Geometry: final body of the model. Coordinates: model frame, mm. A direction names the side the tool comes from. Give positions to 0.01 mm unless a question says otherwise; leave off trailing zeros. Loops run counter-clockwise (first coordinate to the right, second up) from the corner with the lowest first, then second, coordinate; pieces in that order, holes last. Notation, with made-up numbers: (-9, -27.75) - (23, -27.75) arc R16 ccw to (23, -15.75) - close; hole circle Ø3 at (77, 53.5). An arc over 180 degrees is marked (long way). Answer in a Markdown table with one row per item.
from build123d import *

# Parameters (mm, degrees)
EXTRUDE_1_DEPTH     = 2.5
SKETCH_2_R          = 1.6
CUT_EXTRUDE_1_DEPTH = 139.744369255
SKETCH_3_R          = 1.05
CUT_EXTRUDE_2_DEPTH = 139.744369255
SKETCH_4_R          = 1.1
SKETCH_4_R_2        = 15
SKETCH_4_R_3        = 6
CUT_EXTRUDE_3_DEPTH = 139.744369255
CHAMFER_1_SIZE      = 1
CHAMFER_2_SIZE      = 1


with BuildPart() as part:
    # 草图1 → 凸台-拉伸1 (new, symmetric)
    with BuildSketch(Plane.XY):
        with BuildLine():
            Line((-125, 29), (-125, 20))
            ThreePointArc((-125, 20), (-123.535533906, 16.464466094), (-120, 15))
            Line((-120, 15), (-98, 15))
            ThreePointArc((-98, 15), (-94.464466094, 13.535533906), (-93, 10))
            Line((-93, 10), (-93, -10))
            ThreePointArc((-93, -10), (-94.464466094, -13.535533906), (-98, -15))
            Line((-98, -15), (-120, -15))
            ThreePointArc((-120, -15), (-123.535533906, -16.464466094), (-125, -20))
            Line((-125, -20), (-125, -29))
            ThreePointArc((-125, -29), (-124.906679931, -29.9615051), (-124.630203177, -30.88711911))
            Line((-124.630203177, -30.88711911), (-118.51669464, -45.88711911))
            ThreePointArc((-118.51669464, -45.88711911), (-99.99588193, -58.338642669), (-81.475069221, -45.88711911))
            Line((-81.475069221, -45.88711911), (-75.361560684, -30.88711911))
            ThreePointArc((-75.361560684, -30.88711911), (-74.837036555, -30.24239728), (-74.04203004, -30))
            Line((-74.04203004, -30), (-1.339745962, -30))
            ThreePointArc((-1.339745962, -30), (-0.045650737, -30.170370869), (1.160254038, -30.669872981))
            Line((1.160254038, -30.669872981), (50.801270189, -59.330127019))
            ThreePointArc((50.801270189, -59.330127019), (52.007174964, -59.829629131), (53.301270189, -60))
            Line((53.301270189, -60), (95, -60))
            ThreePointArc((95, -60), (98.535533906, -58.535533906), (100, -55))
            Line((100, -55), (100, -32.886751346))
            ThreePointArc((100, -32.886751346), (99.330127019, -30.386751346), (97.5, -28.556624327))
            Line((97.5, -28.556624327), (55.538475773, -4.330127019))
            ThreePointArc((55.538475773, -4.330127019), (53.038475773, 0), (55.538475773, 4.330127019))
            Line((55.538475773, 4.330127019), (97.5, 28.556624327))
            ThreePointArc((97.5, 28.556624327), (99.330127019, 30.386751346), (100, 32.886751346))
            Line((100, 32.886751346), (100, 55))
            ThreePointArc((100, 55), (98.535533906, 58.535533906), (95, 60))
            Line((95, 60), (53.301270189, 60))
            ThreePointArc((53.301270189, 60), (52.007174964, 59.829629131), (50.801270189, 59.330127019))
            Line((50.801270189, 59.330127019), (0, 30))
            Line((0, 30), (-74.04203004, 30))
            ThreePointArc((-74.04203004, 30), (-74.837036555, 30.24239728), (-75.361560684, 30.88711911))
            Line((-75.361560684, 30.88711911), (-81.475069221, 45.88711911))
            ThreePointArc((-81.475069221, 45.88711911), (-99.99588193, 58.338642669), (-118.51669464, 45.88711911))
            Line((-118.51669464, 45.88711911), (-124.630203177, 30.88711911))
            ThreePointArc((-124.630203177, 30.88711911), (-124.906679931, 29.9615051), (-125, 29))
        make_face()
    extrude(amount=EXTRUDE_1_DEPTH, both=True)

    # 草图2 → 切除-拉伸1 (cut, through all)
    with BuildSketch(Plane.XY.offset(2.5)):
        with Locations((-104.99588193, 40)):
            Circle(SKETCH_2_R)
        with Locations((-94.99588193, 40)):
            Circle(SKETCH_2_R)
        with Locations(Location((-94.99588193, -40, 0), (0, 0, 180))):
            Circle(SKETCH_2_R)
        with Locations(Location((-104.99588193, -40, 0), (0, 0, 180))):
            Circle(SKETCH_2_R)
        with Locations((-104.99588193, 30)):
            Circle(SKETCH_2_R)
        with Locations((-94.99588193, 30)):
            Circle(SKETCH_2_R)
        with Locations(Location((-94.99588193, -30, 0), (0, 0, 180))):
            Circle(SKETCH_2_R)
        with Locations(Location((-104.99588193, -30, 0), (0, 0, 180))):
            Circle(SKETCH_2_R)
        with Locations((-94.99588193, 50)):
            Circle(SKETCH_2_R)
        with Locations(Location((-94.99588193, -50, 0), (0, 0, 180))):
            Circle(SKETCH_2_R)
    extrude(amount=-CUT_EXTRUDE_1_DEPTH, mode=Mode.SUBTRACT)

    # 草图3 → 切除-拉伸2 (cut, through all)
    with BuildSketch(Plane.XY.offset(2.5)):
        with Locations((65, 51.1)):
            Circle(SKETCH_3_R)
        with Locations((72, 44.1)):
            Circle(SKETCH_3_R)
        with Locations((58, 44.1)):
            Circle(SKETCH_3_R)
        with Locations((65, 37.1)):
            Circle(SKETCH_3_R)
        with Locations(Location((65, -37.1, 0), (0, 0, 180))):
            Circle(SKETCH_3_R)
        with Locations(Location((58, -44.1, 0), (0, 0, 180))):
            Circle(SKETCH_3_R)
        with Locations(Location((72, -44.1, 0), (0, 0, 180))):
            Circle(SKETCH_3_R)
        with Locations(Location((65, -51.1, 0), (0, 0, 180))):
            Circle(SKETCH_3_R)
    extrude(amount=-CUT_EXTRUDE_2_DEPTH, mode=Mode.SUBTRACT)

    # 草图4 → 切除-拉伸3 (cut, through all)
    with BuildSketch(Plane.XY.offset(2.5)):
        with Locations((-65.894, 24.476)):
            Circle(SKETCH_4_R)
        with Locations((-65.894, -24.476)):
            Circle(SKETCH_4_R)
        with Locations((-8, -24.476)):
            Circle(SKETCH_4_R)
        with Locations((-8, 24.476)):
            Circle(SKETCH_4_R)
        with Locations((-36.947, 0)):
            Circle(SKETCH_4_R_2)
        with Locations((30, 25)):
            Circle(SKETCH_4_R_3)
        with Locations((30, -25)):
            Circle(SKETCH_4_R_3)
    extrude(amount=-CUT_EXTRUDE_3_DEPTH, mode=Mode.SUBTRACT)

    # 倒角1
    chamfer_1_edges = [part.edges().sort_by_distance(p)[0] for p in [
        (53.038475773, 0, 2.5),
        (76.519237886, 16.443375673, 2.5),
        (99.330127019, 30.386751346, 2.5),
        (100, 43.943375673, 2.5),
        (98.535533906, 58.535533906, 2.5),
        (74.150635095, 60, 2.5),
        (52.007174964, 59.829629131, 2.5),
        (25.400635095, 44.665063509, 2.5),
        (-123.535533906, 16.464466094, 2.5),
        (-37.02101502, 30, 2.5),
        (-74.837036555, 30.24239728, 2.5),
        (-78.418314952, 38.38711911, 2.5),
        (-99.99588193, 58.338642669, 2.5),
        (-121.573448909, 38.38711911, 2.5),
        (-109, 15, 2.5),
        (-94.464466094, 13.535533906, 2.5),
        (-93, 0, 2.5),
        (-94.464466094, -13.535533906, 2.5),
        (-109, -15, 2.5),
        (-121.573448909, 38.38711911, -2.5),
        (-99.99588193, 58.338642669, -2.5),
        (-78.418314952, 38.38711911, -2.5),
        (-74.837036555, 30.24239728, -2.5),
        (-37.02101502, 30, -2.5),
        (25.400635095, 44.665063509, -2.5),
        (-123.535533906, -16.464466094, 2.5),
        (52.007174964, 59.829629131, -2.5),
        (74.150635095, 60, -2.5),
        (98.535533906, 58.535533906, -2.5),
        (100, 43.943375673, -2.5),
        (99.330127019, 30.386751346, -2.5),
        (76.519237886, 16.443375673, -2.5),
        (53.038475773, 0, -2.5),
        (76.519237886, -16.443375673, -2.5),
        (99.330127019, -30.386751346, -2.5),
        (100, -43.943375673, -2.5),
        (-125, -24.5, 2.5),
        (98.535533906, -58.535533906, -2.5),
        (74.150635095, -60, -2.5),
        (52.007174964, -59.829629131, -2.5),
        (25.980762114, -45, -2.5),
        (-0.045650737, -30.170370869, -2.5),
        (-37.690888001, -30, -2.5),
        (-74.837036555, -30.24239728, -2.5),
        (-78.418314952, -38.38711911, -2.5),
        (-99.99588193, -58.338642669, -2.5),
        (-121.573448909, -38.38711911, -2.5),
        (-124.906679931, -29.9615051, 2.5),
        (-124.906679931, -29.9615051, -2.5),
        (-125, -24.5, -2.5),
        (-123.535533906, -16.464466094, -2.5),
        (-109, -15, -2.5),
        (-94.464466094, -13.535533906, -2.5),
        (-93, 0, -2.5),
        (-94.464466094, 13.535533906, -2.5),
        (-109, 15, -2.5),
        (-123.535533906, 16.464466094, -2.5),
        (-125, 24.5, -2.5),
        (-121.573448909, -38.38711911, 2.5),
        (-124.906679931, 29.9615051, -2.5),
        (-124.906679931, 29.9615051, 2.5),
        (-99.99588193, -58.338642669, 2.5),
        (-78.418314952, -38.38711911, 2.5),
        (-74.837036555, -30.24239728, 2.5),
        (-37.690888001, -30, 2.5),
        (-0.045650737, -30.170370869, 2.5),
        (25.980762114, -45, 2.5),
        (52.007174964, -59.829629131, 2.5),
        (74.150635095, -60, 2.5),
        (98.535533906, -58.535533906, 2.5),
        (100, -43.943375673, 2.5),
        (-125, 24.5, 2.5),
        (99.330127019, -30.386751346, 2.5),
        (76.519237886, -16.443375673, 2.5),
    ]]
    chamfer(chamfer_1_edges, length=CHAMFER_1_SIZE)

    # 倒角2
    chamfer_2_edges = [part.edges().sort_by_distance(p)[0] for p in [
        (24, -25, -2.5),
        (24, -25, 2.5),
        (24, 25, -2.5),
        (24, 25, 2.5),
        (-51.947, 0, -2.5),
        (-51.947, 0, 2.5),
    ]]
    chamfer(chamfer_2_edges, length=CHAMFER_2_SIZE)


solid = part.part
Q1. Draft query along X for faces 6 (the flat face through (-78.83, 38.1, -1.99)), 7 (the conical face through (98.063, 57.996, -2.215)), 8 (the flat face through (-121.616, -38.282, 0.021)), 9 (the flat face through (25.756, 44.87, 0.021)). Return one class per face: pulls with the +X half, pulls with the -X half, needs draft (parallel to the pull), parting line crosses it, or undercut.
Check values:
| item | result |
|---|---|
| face 6 | undercut |
| face 7 | pulls with the +X half |
| face 8 | pulls with the -X half |
| face 9 | undercut |
Q2. Cut plane B-B (x = 68.5). Output: boundary loops of the cut face in (y, z).
Check values:
| item | result |
|---|---|
| outline | (-60, -1.5) - (-59, -2.5) - (-12.97, -2.5) - (-11.81, -1.5) - (-11.81, 1.5) - (-12.97, 2.5) - (-59, 2.5) - (-60, 1.5) - close; (11.81, -1.5) - (12.97, -2.5) - (59, -2.5) - (60, -1.5) - (60, 1.5) - (59, 2.5) - (12.97, 2.5) - (11.81, 1.5) - close |
Q3. Material intervals for line 1 along Y through (x, z) = (30, -0.55); line 2 along Y through (x, z) = (-65, -1.95); line 3 along Y through (x, z) = (-36, 0.9), sorted ascending.
Check values:
| item | result |
|---|---|
| line 1 | -47.32 to -31, -19 to 19, 31 to 47.32 |
| line 2 | -29.55 to -25.12, -23.84 to 23.84, 25.12 to 29.55 |
| line 3 | -30 to -14.97, 14.97 to 30 |
Q4. Cut plane A-A (x = -55.5). Output: boundary loops of the cut face in (y, z).
Check values:
| item | result |
|---|---|
| outline | (-30, -1.5) - (-29, -2.5) - (29, -2.5) - (30, -1.5) - (30, 1.5) - (29, 2.5) - (-29, 2.5) - (-30, 1.5) - close |
Q5. Cut plane D-D (x = 8.5). Output: boundary loops of the cut face in (y, z).
Check values:
| item | result |
|---|---|
| outline | (-34.91, -1.5) - (-33.75, -2.5) - (33.75, -2.5) - (34.91, -1.5) - (34.91, 1.5) - (33.75, 2.5) - (-33.75, 2.5) - (-34.91, 1.5) - close |
Q6. First-contact query: pin 1 (2 mm diameter, centred on x = -43, z = -2, fed in from +Y); pin 2 (2 mm diameter, centred on x = 43, z = -0.5, fed in from -Y); pin 3 (3 mm diameter, centred on x = 45.5, z = -2, fed in from +Y). Flat tips, straight axial feed; report the tip coordinate or a pass-through.
Check values:
| item | result |
|---|---|
| pin 1 | y = 30 |
| pin 2 | y = -55.4 |
| pin 3 | y = 57.09 |
Q7. Cut plane C-C (z = 0.65). Give the number of separate pieces and of enclosed holes in the cut face, and give its area (3 significant figures).
Check values:
| item | result |
|---|---|
| separate pieces | 1 |
| enclosed holes | 25 |
| area | 16,400 mm² |
Q8. Reachability of faces 1 (the flat face through (-78.46, -38.49, 0.02)), 2 (the flat face through (25.88, -44.372, -1.993)), 3 (the cylindrical face through (-95, 14, 0)), 4 (the flat face through (25.89, 44.38, 1.99)), 5 (the conical face through (-123.063, 17.004, -2.215)) from +Z, -Z, +X, -X, +Y, -Y: full face, straight path, thin tool, end or side. Return the list, or none.
Check values:
| item | result |
|---|---|
| face 1 | +Z, -Z, -Y |
| face 2 | -Z, -Y |
| face 3 | +Z, -Z, -X |
| face 4 | +Z, +Y |
| face 5 | -Z, -X |
